Could you check a few things on this drawing? It's one solid part, dimensions in mm from its lowest x, y, z. Give positions to 0.01 mm unless a question says otherwise; leave off trailing zeros. Loops run counter-clockwise (first coordinate to the right, second up) from the corner with the lowest first, then second, coordinate; pieces in that order, holes last.
1. Thinking about a two-plate mould opening in Z: for the marked faces 1 and 2, which applies, +Z half, -Z half, draft (parallel to the pull), parting line (faces both ways), or undercut?
2. I need wall thicknesses on line 1 along X through (y, z) = (2.6, 60); line 2 along Z through (x, y) = (66, 2.65); line 3 along Y through (x, z) = (14, 42). Which ranges of each line are inside material? Lowest first, please.
3. Imagine slicing it at C-C (x = 66.5). List the corners of the cut face in (y, z) for me, plus the area to 3 significant figures.
4. For P1, Ø1.5, axis at x = 48.5, y = 2, coming from the +Z side; P2, Ø2.5, axis at y = 1.5, z = 32, coming from the -X side; P3, Ø10, axis at x = 11.5, z = 11, coming from the -Y side, each with a flat end and sliding along its axis, tell me the tip position at first contact or that it passes through.
5. Imagine slicing it at B-B (z = 55). List the corners of the cut face in (x, y) for me.
6. Imagine slicing it at A-A (y = 1.3). List the corners of the cut face in (x, z) for me, plus the area to 3 significant figures.
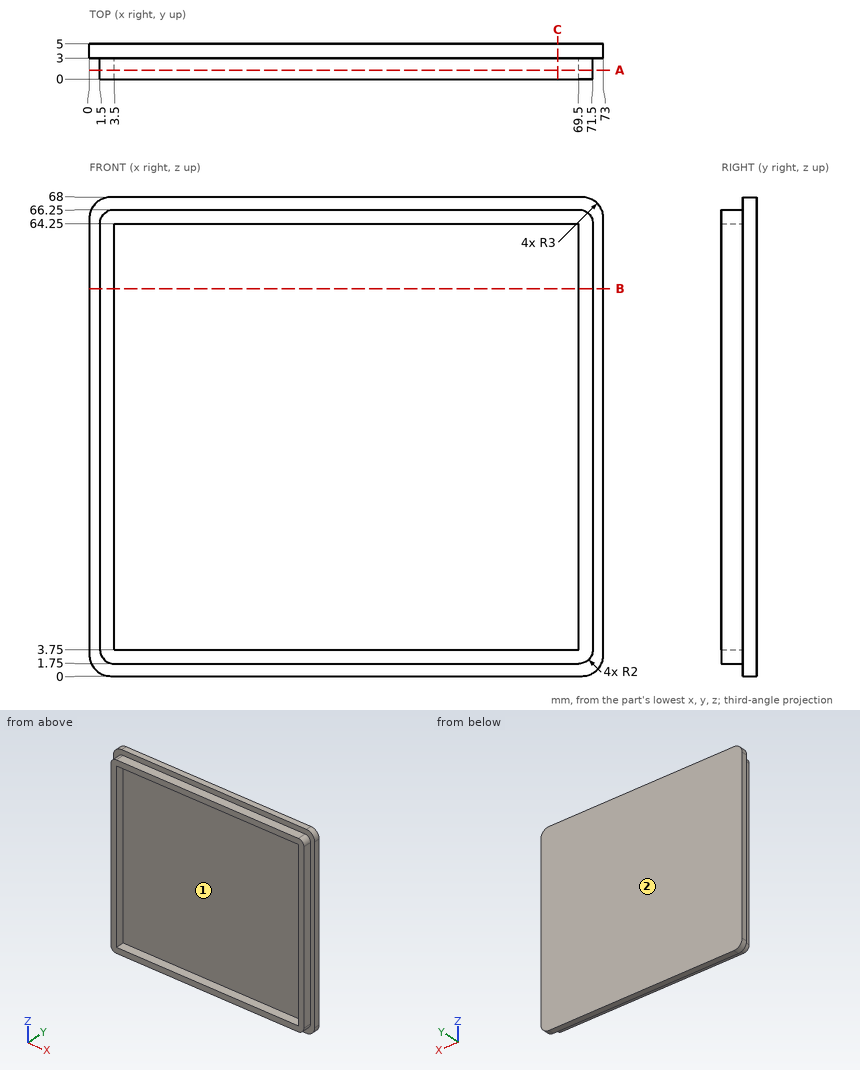
Derived:
1. face 1: undercut
1. face 2: draft
2. line 1: x = 1.5 to 3.5, 69.5 to 71.5
2. line 2: z = 1.75 to 3.75, 64.25 to 66.25
2. line 3: y = 3 to 5
3. outline: (0, 1.75) - (3, 1.75) - (3, 0) - (5, 0) - (5, 68) - (3, 68) - (3, 66.25) - (0, 66.25) - (0, 64.25) - (3, 64.25) - (3, 3.75) - (0, 3.75) - close
3. area: 148 mm2
4. P1: stops at z = 66.25
4. P2: stops at x = 1.5
4. P3: stops at y = 3
5. outline: (0, 3) - (1.5, 3) - (1.5, 0) - (3.5, 0) - (3.5, 3) - (69.5, 3) - (69.5, 0) - (71.5, 0) - (71.5, 3) - (73, 3) - (73, 5) - (0, 5) - close
6. outline: (1.5, 3.75) arc R2 ccw to (3.5, 1.75) - (69.5, 1.75) arc R2 ccw to (71.5, 3.75) - (71.5, 64.25) arc R2 ccw to (69.5, 66.25) - (3.5, 66.25) arc R2 ccw to (1.5, 64.25) - close; hole (3.5, 3.75) - (69.5, 3.75) - (69.5, 64.25) - (3.5, 64.25) - close
6. area: 519 mm2
